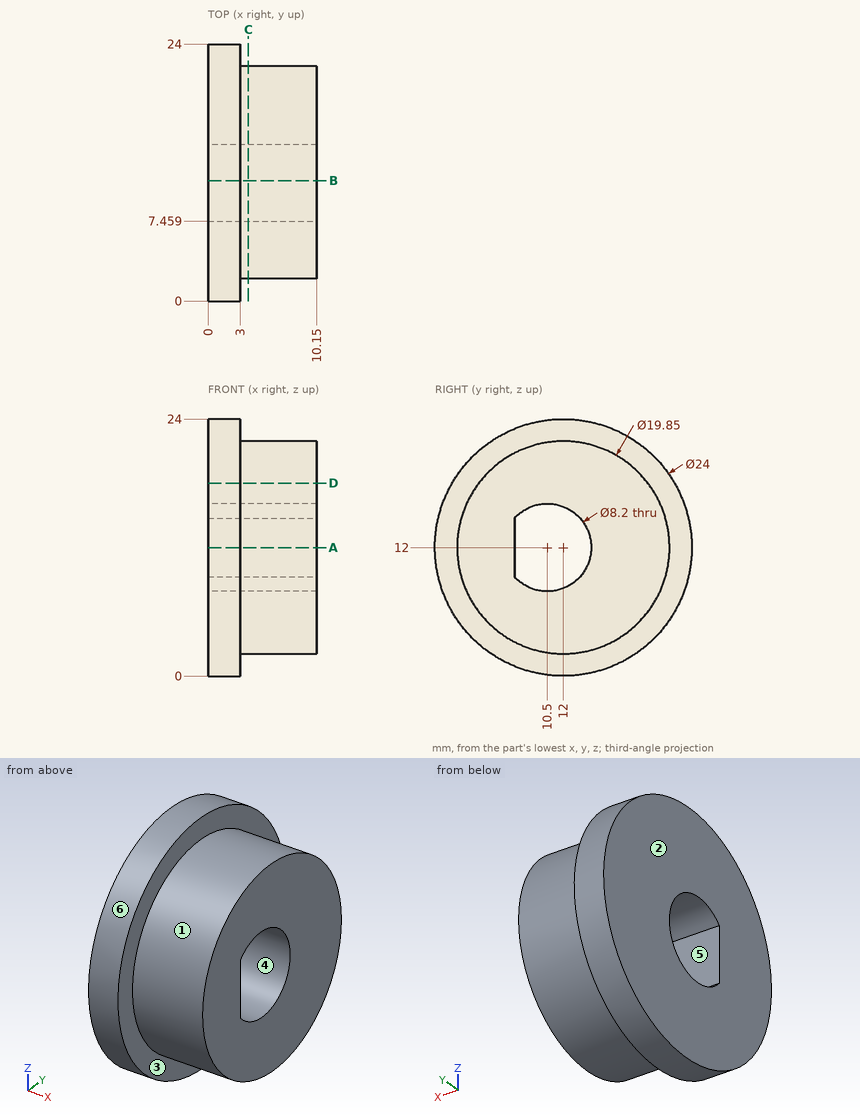
Job drawing, mm, ordinate dimensions from the low corner. One solid piece. A direction names the side the tool comes from. Give positions to 0.01 mm unless a question says otherwise; leave off trailing zeros. Write each loop counter-clockwise with the first axis right and the second up, starting at its lowest first coordinate (ties: lowest second). Pieces come first, ordered by that corner, then holes. Notation, with made-up numbers: (75, 13.25) -> (92, 13.25) arc R35 cw to (92, 48.25) -> close; hole circle Ø4 at (-7, -14). An arc over 180 degrees is marked (long way). Return JSON: item names as keys, results as strings.
Item 1: Tool access for the marked faces 1 and 2: list every direction of +Z, -Z, +X, -X, +Y, -Y with a clear straight run to the whole face (end or side of a thin tool).
Answer below:
{"face 1": "+X", "face 2": "+Z, -Z, -X, +Y, -Y"}
Item 2: Band-saw the part on C-C (x = 3.75). List the corners of the cut face in (y, z) (3 decimals).
Answer below:
{"outline": "circle Ø19.85 at (12, 12); hole (7.459, 9.25) arc R4.1 ccw (long way) to (7.459, 14.75) -> close"}
Item 3: Two-plate mould, pull along Y, no slides. Class the marked faces 3, 4, 5 and 6: +Y half, -Y half, draft (parallel to the pull), parting line (faces both ways), or undercut.
Answer below:
{"face 3": "draft", "face 4": "undercut", "face 5": "undercut", "face 6": "parting line"}
Item 4: Band-saw the part on B-B (y = 11.25). List the corners of the cut face in (x, z).
Answer below:
{"outline": "(0, 0.02) -> (3, 0.02) -> (3, 2.1) -> (10.15, 2.1) -> (10.15, 7.97) -> (0, 7.97) -> close; (0, 16.03) -> (10.15, 16.03) -> (10.15, 21.9) -> (3, 21.9) -> (3, 23.98) -> (0, 23.98) -> close"}
Item 5: Band-saw the part on D-D (z = 18). List the corners of the cut face in (x, y).
Answer below:
{"outline": "(0, 1.61) -> (3, 1.61) -> (3, 4.09) -> (10.15, 4.09) -> (10.15, 19.91) -> (3, 19.91) -> (3, 22.39) -> (0, 22.39) -> close"}
Item 6: Drop flat-ended pins along their axis: pin 1 (1.6 mm diameter, centred on x = 7, z = 13, fed in from +Y); pin 2 (6 mm diameter, centred on x = 6.5, y = 8, fed in from -Z); pin 3 (8 mm diameter, centred on y = 21, z = 10.5, fed in from -X); pin 4 (1 mm diameter, centred on x = 8, y = 3, fed in from -Z). Give the stop position or say it passes through.
Answer below:
{"pin 1": "stops at y = 21.92", "pin 2": "stops at z = 2.13", "pin 3": "stops at x = 0", "pin 4": "stops at z = 6.88"}
Item 7: Drill centre lines: probe 1 along Y at (x, z) = (6, 12) (3 decimals); probe 2 along Z at (x, y) = (7, 9); probe 3 along Y at (x, z) = (4.75, 15.5). Where is each one in solid material? Low to high.
Answer below:
{"probe 1": "y = 2.075 to 7.459, 14.6 to 21.925", "probe 2": "z = 2.54 to 8.18, 15.82 to 21.46", "probe 3": "y = 2.71 to 8.36, 12.64 to 21.29"}
Item 8: Band-saw the part on A-A (z = 12). List the corners of the cut face in (x, y) (3 decimals).
Answer below:
{"outline": "(0, 0) -> (3, 0) -> (3, 2.075) -> (10.15, 2.075) -> (10.15, 7.459) -> (0, 7.459) -> close; (0, 14.6) -> (10.15, 14.6) -> (10.15, 21.925) -> (3, 21.925) -> (3, 24) -> (0, 24) -> close"}
